from build123d import *

# Parameters (mm, degrees)
EXTRUDE_1_DEPTH     = 190
SKETCH_2_R          = 2.25
CUT_EXTRUDE_1_DEPTH = 2
SKETCH_3_R          = 2.25
CUT_EXTRUDE_2_DEPTH = 21


with BuildPart() as part:
    # Эскиз1 → Бобышка-Вытянуть1 (new body)
    with BuildSketch(Plane(origin=(0, 0, 0), x_dir=(1, 0, 0), z_dir=(0, 1, 0))):
        Polygon((0, 0), (0, 20), (1, 20), (1, 1), (20, 1), (20, 0), align=None)
    extrude(amount=EXTRUDE_1_DEPTH)

    # Эскиз2 → Вырез-Вытянуть1 (cut, through all)
    with BuildSketch(Plane(origin=(1, 0, 0), x_dir=(0, 0, -1), z_dir=(1, 0, 0))):
        with Locations((10.5, 10)):
            Circle(SKETCH_2_R)
        with Locations((10.5, 180)):
            Circle(SKETCH_2_R)
    extrude(amount=-CUT_EXTRUDE_1_DEPTH, mode=Mode.SUBTRACT)

    # Эскиз3 → Вырез-Вытянуть2 (cut, through all)
    with BuildSketch(Plane.ZY):
        with Locations((-10.5, 159.5)):
            Circle(SKETCH_3_R)
    extrude(amount=-CUT_EXTRUDE_2_DEPTH, mode=Mode.SUBTRACT)


solid = part.part
Input: part model. Units: mm. Frame: model coordinates. A direction names the side the tool comes from. Give positions to 0.01 mm unless a question says otherwise; leave off trailing zeros. Order: outer loops, then holes, each group sorted by start corner. A loop starts at its lowest first (then second) coordinate and runs counter-clockwise, first axis right, second up. Notation, with made-up numbers: (57, 14) -> (110, 14) arc R18 cw to (110, 46) -> close; hole circle Ø1 at (-33, -3). An arc over 180 degrees is marked (long way). Use one line per item in the form item = value.
1) Reachability of faces 4 (the flat face through (10, 94, -1)), 5 (the cylindrical face through (0.507, 177.804, -10.012)) from +Z, -Z, +X, -X, +Y, -Y: full face, straight path, thin tool, end or side. Return the list, or none.
Response values:
face_4 = -Z, +X, +Y, -Y
face_5 = +X, -X
2) First-contact query: pin 1 Ø10 at (x, z) = (7, -4) entering from -Y; pin 2 Ø1.5 at (y, z) = (167, -17) entering from +X; pin 3 Ø12 at (x, y) = (17.5, 151) entering from -Z; pin 4 Ø3.5 at (y, z) = (180, -10.5) entering from +X. Flat tips, straight axial feed; report the tip coordinate or a pass-through.
Response values:
pin_1 = 0
pin_2 = 1
pin_3 = -1
pin_4 = through
3) Section A-A, the plane y = 180. Return loops of the section in (x, z), and give its area (3 significant figures).
Response values:
outline = (0, -20) -> (1, -20) -> (1, -12.75) -> (0, -12.75) -> close; (0, -8.25) -> (1, -8.25) -> (1, -1) -> (20, -1) -> (20, 0) -> (0, 0) -> close
area = 34.5 mm^2
4) Section B-B, the plane z = -10.5. Return loops of the section in (x, y), and give its area (4 significant figures).
Response values:
outline = (0, 0) -> (1, 0) -> (1, 7.75) -> (0, 7.75) -> close; (0, 12.25) -> (1, 12.25) -> (1, 157.25) -> (0, 157.25) -> close; (0, 161.75) -> (1, 161.75) -> (1, 177.75) -> (0, 177.75) -> close; (0, 182.25) -> (1, 182.25) -> (1, 190) -> (0, 190) -> close
area = 176.5 mm^2
5) Section C-C, the plane y = 92. Return loops of the section in (x, z), and give its area (3 significant figures).
Response values:
outline = (0, -20) -> (1, -20) -> (1, -1) -> (20, -1) -> (20, 0) -> (0, 0) -> close
area = 39.0 mm^2
6) Mould query, pull axis Y, two halves, no side actions, for faces 1 (the flat face through (0, 94, -10)), 2 (the cylindrical face through (0.51, 11.52, -8.84)), 3 (the flat face through (5.6, 0, -0.4)). Classes: pulls with the +Y half, pulls with the -Y half, needs draft (parallel to the pull), parting line crosses it, or undercut.
Response values:
face_1 = needs draft
face_2 = undercut
face_3 = pulls with the -Y half
7) Line query: probe 1 along Y at (x, z) = (0.3, -10.5); probe 2 along Z at (x, y) = (0.75, 159.5); probe 3 along X at (y, z) = (159, -2.5). Output: solid intervals per line, ascending.
Response values:
probe_1 = 0 to 7.75, 12.25 to 157.25, 161.75 to 177.75, 182.25 to 190
probe_2 = -20 to -12.75, -8.25 to 0
probe_3 = 0 to 1
8) Section D-D, the plane x = 15.5. Return loops of the section in (y, z), and give its area (3 significant figures).
Response values:
outline = (0, -1) -> (190, -1) -> (190, 0) -> (0, 0) -> close
area = 190 mm^2
